Work out the finished part from the listing and answer in its coordinate system (mm). Face numbers are marked on the shaded views. A direction names the side the tool comes from. Round coordinates to 2 decimals unless told otherwise and drop trailing zeros. Write each loop counter-clockwise with the first axis right and the second up, starting at its lowest first coordinate (ties: lowest second). Pieces come first, ordered by that corner, then holes.
1. Find section A-A (z = 105.92). Write down the section's boundary in (x, y), and give its area (3 significant figures).
2. Find section C-C (z = 147.94). Write down the section's boundary in (x, y), and give its area (3 significant figures).
3. A tool of negligible diameter and unlimited length cuts with its end or side. For the marked faces 1, 2, 3 and 4, from which of +Z, -Z, +X, -X, +Y, -Y can it reach the whole face along a straight path? Write none if from no direction.
4. Find section D-D (x = 19). Write down the section's boundary in (y, z), and give its area (3 significant figures).
5. Flat-ended cylindrical pins translate along their axes: pin 1 Ø6 at (x, z) = (19.5, 113.5) entering from +Y; pin 2 Ø17.5 at (x, z) = (4.5, 103.5) entering from -Y; pin 3 Ø0.9 at (x, y) = (-0.5, 24) entering from +Z. Find the tip coordinate at first contact, or state that the pin passes through.
6. Straight lines are drawn through the part: probe 1 along X at (y, z) = (-9.5, 91.93); probe 2 along Y at (x, z) = (9.5, 113); probe 3 along X at (y, z) = (-4, 91). For each, find the intervals that lie inside material, in ascending order.
7. Find section B-B (y = 0). Write down the section's boundary in (x, z), and give its area (3 significant figures).
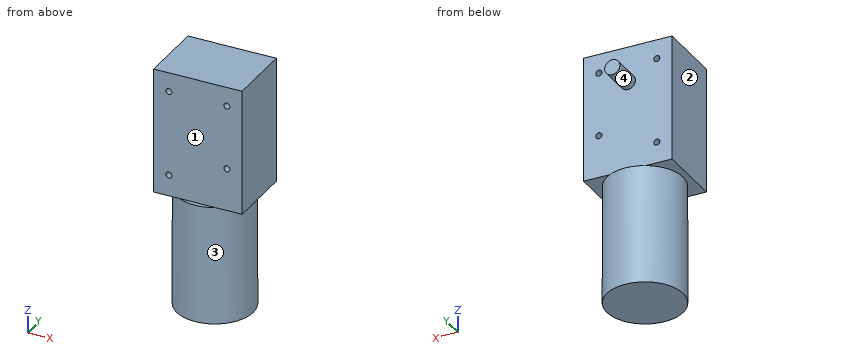
```python
from build123d import *

# Parameters (mm, degrees)
SKETCH1_R           = 25
BOSS_EXTRUDE1_DEPTH = 78
SKETCH2_W           = 58
SKETCH2_H           = 44
BOSS_EXTRUDE2_DEPTH = 82.5
SKETCH3_R           = 5
BOSS_EXTRUDE3_DEPTH = 20
SKETCH4_R           = 2
CUT_EXTRUDE1_DEPTH  = 170.73582415


with BuildPart() as part:
    # Sketch1 → Boss-Extrude1 (new body)
    with BuildSketch(Plane.XY):
        Circle(SKETCH1_R)
    extrude(amount=BOSS_EXTRUDE1_DEPTH)

    # Sketch2 → Boss-Extrude2 (add)
    with BuildSketch(Plane.XY.offset(78)):
        Rectangle(SKETCH2_W, SKETCH2_H)
    extrude(amount=BOSS_EXTRUDE2_DEPTH)

    # Sketch3 → Boss-Extrude3 (add)
    with BuildSketch(Plane(origin=(0, 22, 0), x_dir=(1, 0, 0), z_dir=(0, 1, 0))):
        with Locations(Location((0, -137, 0), (0, 0, 270))):
            Circle(SKETCH3_R)
    extrude(amount=BOSS_EXTRUDE3_DEPTH)

    # Sketch4 → Cut-Extrude1 (cut, through all)
    with BuildSketch(Plane(origin=(0, 22, 0), x_dir=(1, 0, 0), z_dir=(0, 1, 0))):
        with Locations(Location((19, -147.94, 0), (0, 0, 270))):
            Circle(SKETCH4_R)
        with Locations(Location((19, -105.92, 0), (0, 0, 270))):
            Circle(SKETCH4_R)
        with Locations(Location((-19, -147.94, 0), (0, 0, 270))):
            Circle(SKETCH4_R)
        with Locations(Location((-19, -91.93, 0), (0, 0, 270))):
            Circle(SKETCH4_R)
    extrude(amount=-CUT_EXTRUDE1_DEPTH, mode=Mode.SUBTRACT)


solid = part.part
```
Worked answers:
1. outline: (-29, -22) - (17, -22) - (17, 22) - (-29, 22) - close; (21, -22) - (29, -22) - (29, 22) - (21, 22) - close
1. area: 2,380 mm2
2. outline: (-29, -22) - (-21, -22) - (-21, 22) - (-29, 22) - close; (-17, -22) - (17, -22) - (17, 22) - (-17, 22) - close; (21, -22) - (29, -22) - (29, 22) - (21, 22) - close
2. area: 2,200 mm2
3. face 1: +Z, +X, -X, -Y
3. face 2: +Z, -Z, -X, +Y, -Y
3. face 3: -Z
3. face 4: +Y
4. outline: (-22, 78) - (-16.25, 78) - (-16.25, 0) - (16.25, 0) - (16.25, 78) - (22, 78) - (22, 103.92) - (-22, 103.92) - close; (-22, 107.92) - (22, 107.92) - (22, 145.94) - (-22, 145.94) - close; (-22, 149.94) - (22, 149.94) - (22, 160.5) - (-22, 160.5) - close
4. area: 5,810 mm2
5. pin 1: stops at y = 22
5. pin 2: stops at y = -22
5. pin 3: stops at z = 142
6. probe 1: x = -29 to -21, -17 to 29
6. probe 2: y = -22 to 22
6. probe 3: x = -29 to -20.77, -17.23 to 29
7. outline: (-29, 78) - (-25, 78) - (-25, 0) - (25, 0) - (25, 78) - (29, 78) - (29, 160.5) - (-29, 160.5) - close; hole circle Ø4 at (-19, 91.93); hole circle Ø4 at (-19, 147.94); hole circle Ø4 at (19, 105.92); hole circle Ø4 at (19, 147.94)
7. area: 8,630 mm2
